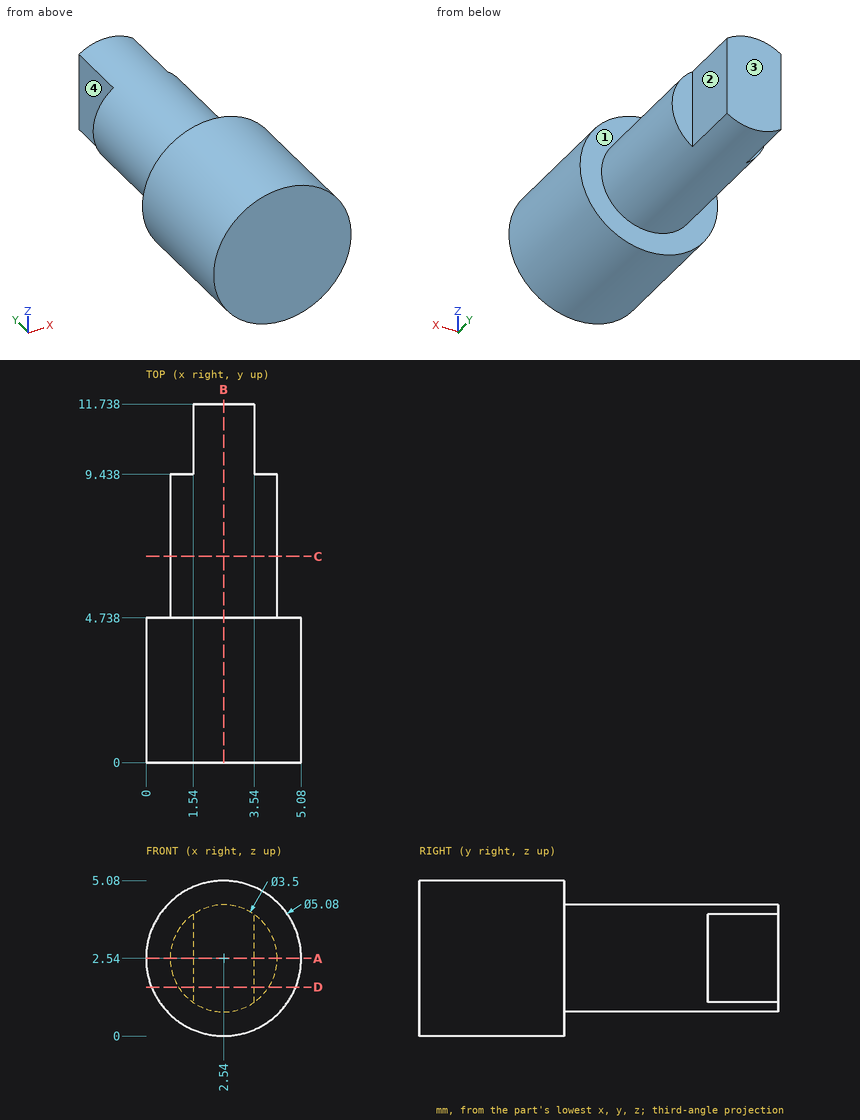
Input: dimensioned drawing with shaded views. Units: mm. Origin: part minimum x, y, z. A direction names the side the tool comes from. Round coordinates to 2 decimals unless told otherwise and drop trailing zeros. Loops run counter-clockwise (first coordinate to the right, second up) from the corner with the lowest first, then second, coordinate; pieces in that order, holes last. Notation, with made-up numbers: M 52,16 L 106,16 A28 cw 106,48 Z; hole C 89.25,-23.75 d11. An arc over 180 degrees is marked long. One line per question, with ' | ' between items.
(1) Material intervals for line 1 along Z through (x, y) = (2.65, 4); line 2 along Y through (x, z) = (4.55, 2.45); line 3 along Y through (x, z) = (3.9, 2.5), sorted ascending. Write a range as from..to.
Check result:
line 1: z = 0..5.08 | line 2: y = 0..4.74 | line 3: y = 0..9.44
(2) Cut plane A-A on z = 2.54. Return the cut outline in (x, y).
Check result:
outline: M 0,0 L 5.08,0 L 5.08,4.74 L 4.29,4.74 L 4.29,9.44 L 3.54,9.44 L 3.54,11.74 L 1.54,11.74 L 1.54,9.44 L 0.79,9.44 L 0.79,4.74 L 0,4.74 Z
(3) Cut plane B-B on x = 2.54. Return the cut outline in (y, z), plus the area to 3 significant figures.
Check result:
outline: M 0,0 L 4.74,0 L 4.74,0.79 L 11.74,0.79 L 11.74,4.29 L 4.74,4.29 L 4.74,5.08 L 0,5.08 Z | area: 48.6 mm2
(4) Cut plane C-C on y = 6.75. Return the cut outline in (x, z).
Check result:
outline: C 2.54,2.54 d3.5
(5) Cut plane D-D on z = 1.6. Return the cut outline in (x, y), plus the area to 3 significant figures.
Check result:
outline: M 0.18,0 L 4.9,0 L 4.9,4.74 L 4.02,4.74 L 4.02,9.44 L 3.54,9.44 L 3.54,11.74 L 1.54,11.74 L 1.54,9.44 L 1.06,9.44 L 1.06,4.74 L 0.18,4.74 Z | area: 40.8 mm2
(6) Contact query for flat-ended pins moving along their axis: P1, Ø0.7, axis at y = 11, z = 2.5, coming from the +X side; P2, Ø2, axis at x = 4, y = 4, coming from the -Z side; P3, Ø0.6, axis at x = 4, z = 2, coming from the +Y side. Output: stop coordinate, or through.
Check result:
P1: stops at x = 3.54 | P2: stops at z = 0.04 | P3: stops at y = 9.44
(7) Access query for the marked faces 1, 2, 3 and 4. Directions: +Z, -Z, +X, -X, +Y, -Y. A direction counts if a zero-diameter tool reaches every point of the face in a straight line with its end or side. Return the directions, or none.
Check result:
face 1: +Y | face 2: +Z, -Z, +X, +Y | face 3: +Z, -Z, +X, -X, +Y | face 4: +Z, -Z, -X, +Y
